Geometry: final body of the model. Coordinates: model frame, mm. Give positions to 0.01 mm unless a question says otherwise; leave off trailing zeros. Write each loop counter-clockwise with the first axis right and the second up, starting at its lowest first coordinate (ties: lowest second). Pieces come first, ordered by that corner, then holes. Notation, with made-up numbers: M 0,9.25 L 7,9.25 A17 cw 7,18.25 Z; hole C 28.5,38 d11. An arc over 180 degrees is marked long. One line per question, with ' | ' between items.
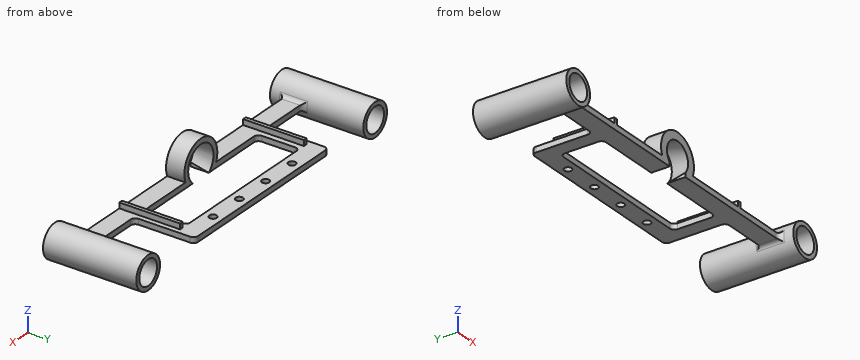
from build123d import *

# Parameters (mm, degrees)
BOSS_EXTRUDE1_DEPTH      = 38.1
BOSS_EXTRUDE1_DEPTH_BACK = 12.7
SKETCH1_R                = 9
SKETCH2_R                = 6.75
CUT_EXTRUDE1_DEPTH       = 50.8
BOSS_EXTRUDE2_DEPTH      = 1.5
BOSS_EXTRUDE2_DEPTH_BACK = 1.5
BOSS_EXTRUDE3_DEPTH      = 10
SKETCH9_W                = 12.009184536
SKETCH9_H                = 15.938825618
CUT_EXTRUDE2_DEPTH       = 3
SKETCH10_R               = 2
CUT_EXTRUDE3_DEPTH       = 3
SKETCH11_W               = 2
SKETCH11_H               = 33.1
BOSS_EXTRUDE4_DEPTH      = 3
FILLET1_R                = 2.5


with BuildPart() as part:
    # Sketch1 → Boss-Extrude1 (new, two sides: drawn at the far end of the back side and taken through both)
    with BuildSketch(Plane(origin=(0, 0, 0), x_dir=(1, 0, 0), z_dir=(0, 1, 0)).offset(-BOSS_EXTRUDE1_DEPTH_BACK)):
        with Locations(Location((86.2, 0, 0), (0, 0, 270))):
            Circle(SKETCH1_R)
    extrude(amount=BOSS_EXTRUDE1_DEPTH + BOSS_EXTRUDE1_DEPTH_BACK)

    # Sketch2 → Cut-Extrude1 (cut)
    with BuildSketch(Plane(origin=(0, -12.7, 0), x_dir=(-1, 0, 0), z_dir=(0, -1, 0))):
        with Locations(Location((-86.2, 0, 0), (0, 0, 90))):
            Circle(SKETCH2_R)
    extrude(amount=-CUT_EXTRUDE1_DEPTH, mode=Mode.SUBTRACT)

    # Sketch4 → Boss-Extrude2 (add, two sides: drawn at the far end of the back side and taken through both)
    with BuildSketch(Plane.XY.offset(-BOSS_EXTRUDE2_DEPTH_BACK)):
        Polygon((77.5, -5), (0, -5), (0, 5), (42.8, 5), (42.8, 28.1), (0, 28.1), (0, 38.1), (50.8, 38.1), (50.8, 28.1), (50.8, 5), (77.5, 5), align=None)
    extrude(amount=BOSS_EXTRUDE2_DEPTH + BOSS_EXTRUDE2_DEPTH_BACK)

    # Mirror2: part across plane


with BuildPart() as part_1:
    add(part.part)
    add(part.part.mirror(Plane(origin=(0, 38.1, -1.5), x_dir=(0, 0, 1), z_dir=(-1, 0, 0))))

    # Sketch6 → Boss-Extrude3 (add)
    with BuildSketch(Plane.XZ.offset(5)):
        with BuildLine():
            Line((10, -1.5), (-10, -1.5))
            ThreePointArc((-10, -1.5), (0, 18.5), (10, -1.5))
        make_face()
    extrude(amount=-BOSS_EXTRUDE3_DEPTH)

    # Cut-Loft1: read off the stored shape, not the designer's step
    # Cut-Loft1: loft between two sections, ruled curve by curve
    cut_loft1_from = [
        Edge.make_bspline([(-6.970459828, 5, 12.611945372), (-20.194350572, 5, -1.328974284), (-6.253430916, 5, -14.552865027), (6.970459828, 5, -0.611945372), (20.194350572, 5, 13.328974284), (6.253430916, 5, 26.552865027), (-6.970459828, 5, 12.611945372)], [0, 0, 0, 0, 0.5, 0.5, 0.5, 1, 1, 1, 1], 3, [1, 0.333333333, 0.333333333, 1, 0.333333333, 0.333333333, 1]),
    ]
    cut_loft1_to = [
        Edge.make_bspline([(-4.235564338, -5, 12.786751413), (-17.809067164, -5, 4.315622738), (-9.337938488, -5, -9.257880088), (4.235564338, -5, -0.786751413), (17.809067164, -5, 7.684377262), (9.337938488, -5, 21.257880088), (-4.235564338, -5, 12.786751413)], [0, 0, 0, 0, 0.5, 0.5, 0.5, 1, 1, 1, 1], 3, [1, 0.333333333, 0.333333333, 1, 0.333333333, 0.333333333, 1]),
    ]
    cut_loft1 = Solid(Shell([*[Face.make_surface_from_curves(cut_loft1_from[k], cut_loft1_to[k]) for k in range(1)], Face(Wire(cut_loft1_from)), Face(Wire(cut_loft1_to))]))
    add(cut_loft1, mode=Mode.SUBTRACT)

    # Sketch9 → Cut-Extrude2 (cut)
    with BuildSketch(Plane(origin=(0, 0, -1.5), x_dir=(-1, 0, 0), z_dir=(0, 0, -1))):
        with Locations((-2.92e-07, -2.969412809)):
            Rectangle(SKETCH9_W, SKETCH9_H)
    extrude(amount=-CUT_EXTRUDE2_DEPTH, mode=Mode.SUBTRACT)

    # Sketch10 → Cut-Extrude3 (cut)
    with BuildSketch(Plane.XY.offset(1.5)):
        with Locations((-30, 33.1)):
            Circle(SKETCH10_R)
        with Locations((-10, 33.1)):
            Circle(SKETCH10_R)
        with Locations((10, 33.1)):
            Circle(SKETCH10_R)
        with Locations((30, 33.1)):
            Circle(SKETCH10_R)
    extrude(amount=-CUT_EXTRUDE3_DEPTH, mode=Mode.SUBTRACT)

    # Sketch11 → Boss-Extrude4 (add)
    with BuildSketch(Plane.XY.offset(1.5)):
        with Locations((-47, 11.55)):
            Rectangle(SKETCH11_W, SKETCH11_H)
        with Locations((47, 11.55)):
            Rectangle(SKETCH11_W, SKETCH11_H)
    extrude(amount=BOSS_EXTRUDE4_DEPTH)

    # Fillet1
    fillet1_edges = [part_1.edges().sort_by_distance(p)[0] for p in [
        (50.8, 5, 0),
        (-50.8, 5, 0),
        (-42.8, 5, 0),
        (-42.8, 28.1, 0),
        (42.8, 5, 0),
        (42.8, 28.1, 0),
        (-77.325880325, 0, -1.5),
        (-77.325880325, 0, 1.5),
        (-77.2, -5, 0),
        (-77.2, 5, 0),
        (77.325880325, 0, -1.5),
        (77.2, -5, 0),
        (77.325880325, 0, 1.5),
        (77.2, 5, 0),
        (50.8, 38.1, 0),
        (-50.8, 38.1, 0),
    ]]
    fillet(fillet1_edges, radius=FILLET1_R)


solid = part_1.part
(1) Cut plane D-D, the plane y = -3. Count the separate pieces of the cut face and the enclosed holes in it, then the cut area to 3 significant figures.
Working result:
separate pieces: 1 | enclosed holes: 2 | area: 841 mm^2
(2) First-contact query: P1, Ø1, axis at x = -61, y = -3.5, coming from the -Z side; P2, Ø3.5, axis at x = -59.5, z = 0.5, coming from the +Y side; P3, Ø2, axis at y = 4.5, z = 9, coming from the +X side; P4, Ø10, axis at y = 21, z = 5, coming from the -X side. Flat tips, straight axial feed; report the tip coordinate or a pass-through.
Working result:
P1: stops at z = -1.5 | P2: stops at y = 5 | P3: stops at x = 90.32 | P4: stops at x = -95.2
(3) Material intervals for L1, parallel to Y at x = 30, z = 0.7; L2, parallel to X at y = 15, z = 0; L3, parallel to Z at x = -86.2, y = 27.5, sorted ascending. Write a range as [from, to].
Working result:
L1: y = [-5, 5], [28.1, 31.1], [35.1, 38.1] | L2: x = [-95.2, -92.95], [-79.45, -77.2], [-50.8, -42.8], [42.8, 50.8], [77.2, 79.45], [92.95, 95.2] | L3: z = [-9, -6.75], [6.75, 9]
(4) Cut plane A-A, the plane y = 19.5. Return loops of the section in (x, z), then the cut area to 3 significant figures.
Working result:
outline: C -86.2,0 d18; M -50.8,-1.5 L -42.8,-1.5 L -42.8,1.5 L -46,1.5 L -46,4.5 L -48,4.5 L -48,1.5 L -50.8,1.5 Z; M 42.8,-1.5 L 50.8,-1.5 L 50.8,1.5 L 48,1.5 L 48,4.5 L 46,4.5 L 46,1.5 L 42.8,1.5 Z; C 86.2,0 d18; hole C -86.2,0 d13.5; hole C 86.2,0 d13.5 | area: 283 mm^2
(5) Cut plane C-C, the plane x = 86.2. Return loops of the section in (y, z), then the cut area to 3 significant figures.
Working result:
outline: M -12.7,-9 L 38.1,-9 L 38.1,-6.75 L -12.7,-6.75 Z; M -12.7,6.75 L 38.1,6.75 L 38.1,9 L -12.7,9 Z | area: 229 mm^2
(6) Cut plane B-B, the plane x = -30. Return loops of the section in (y, z), then the cut area to 3 significant figures.
Working result:
outline: M -5,-1.5 L 5,-1.5 L 5,1.5 L -5,1.5 Z; M 28.1,-1.5 L 31.1,-1.5 L 31.1,1.5 L 28.1,1.5 Z; M 35.1,-1.5 L 38.1,-1.5 L 38.1,1.5 L 35.1,1.5 Z | area: 48.0 mm^2
